Can you work these out from the model? Positions are in its coordinate system, mm. A direction names the side the tool comes from. Round coordinates to 2 decimals unless told otherwise and drop trailing zeros. Loops run counter-clockwise (first coordinate to the right, second up) from the corner with the lowest first, then second, coordinate; pieces in that order, holes last.
(1) I want a section at A-A on z = 16.5. Write out the boundary of the cut face in (x, y).
(2) Will these pins go through, and if not, where does the flat tip stop? pin 1 Ø1 at (x, z) = (0, 19) entering from +Y; pin 2 Ø1.8 at (x, y) = (-0.5, 0.5) entering from -Z; pin 3 Ø3 at (x, z) = (-1, 7.5) entering from -Y; pin 4 Ø1.5 at (y, z) = (-1, 4) entering from +X.
(3) Which directions (+Z, -Z, +X, -X, +Y, -Y) give clear straight access to the entire face, cutting with the end or side of a thin tool? Please do faces 1 (the face through (0, 0, 0)), 2 (the face through (1, -2, 24)).
(4) If I drill on line 1 along Y through (x, z) = (0, 11.25); line 2 along Y through (x, z) = (1.75, 4); line 3 along Z through (x, y) = (-0.5, -2), over which ranges is the centre line in solid material (lowest first)?
Autodesk Inventor part; units mm, degrees
ref_plane "YZ Plane" through (0, 0, 0) normal (1, 0, 0) x (0, 1, 0)
ref_plane "XZ Plane" through (0, 0, 0) normal (0, 1, 0) x (-1, 0, 0)
ref_plane "XY Plane" through (0, 0, 0) normal (0, 0, 1) x (1, 0, 0)
sketch "スケッチ1" plane through (0, 0, 0) normal (0, 0, 1) x (1, 0, 0)
  circle A0 centre (0, 0) radius 2
  dimension "d0" = 4
extrude "押し出し1" add sketch "スケッチ1" along normal blind 24
sketch "スケッチ2" plane through (0, 0, 24) normal (0, 0, 1) x (1, 0, 0)
  circle A0 centre (0, 0) radius 2
  circle A1 centre (0, 0) radius 3
  dimension "d3" = 6
extrude "押し出し2" add sketch "スケッチ2" along normal blind 2 contours A0 | A1
fillet "フィレット1" radius 2 1 edges at (-3, 0, 26)
properties part number "M4ボタンボルト24" material "鋼、高強度、低合金"
Filled sheet:
1. outline: circle Ø4 at (0, 0)
2. pin 1: stops at y = 2
2. pin 2: stops at z = 0
2. pin 3: stops at y = -2
2. pin 4: stops at x = 1.98
3. face 1: -Z, +X, -X, +Y, -Y
3. face 2: -Z
4. line 1: y = -2 to 2
4. line 2: y = -0.97 to 0.97
4. line 3: z = 24 to 25.7
